Design review of the part shown in the three views and the two pictorial views. Dimensions are in mm from the part's minimum x, y and z. Round coordinates to 2 decimals unless told otherwise and drop trailing zeros. Order: outer loops, then holes, each group sorted by start corner. A loop starts at its lowest first (then second) coordinate and runs counter-clockwise, first axis right, second up. Notation, with made-up numbers: (-23.5, -0.5) - (30.5, -0.5) arc R24 ccw to (30.5, 18.5) - close; hole circle Ø8 at (30, 58). An arc over 180 degrees is marked (long way). Use CSV: the item, a comma, the result in double quotes.
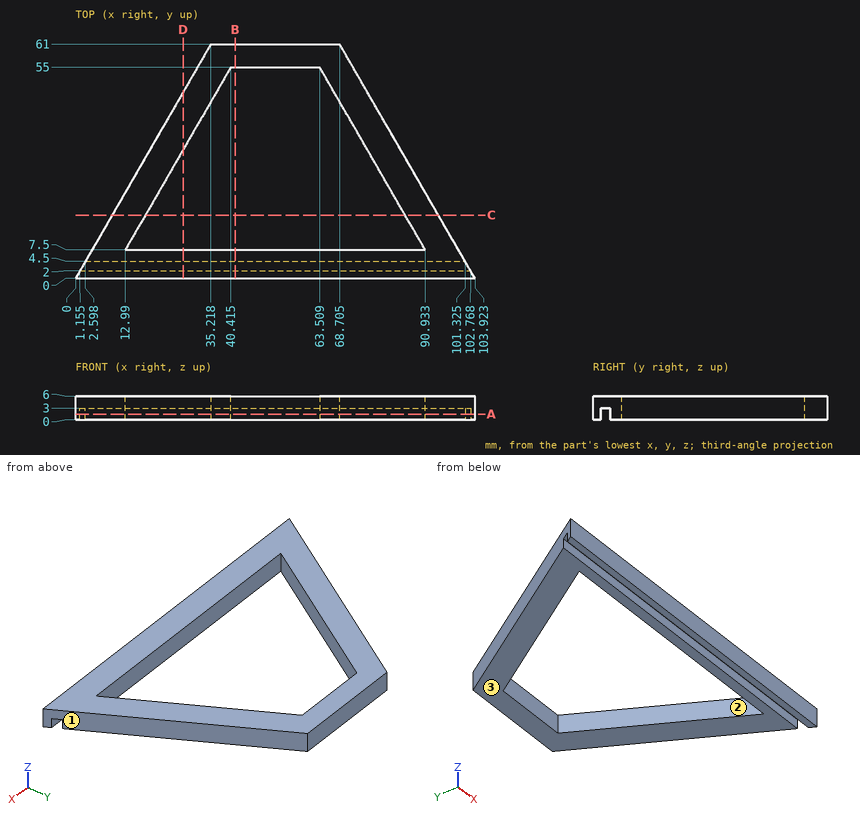
1) We need section B-B (x = 41.5). Give the boundary of the cut face in (y, z).
Data:
outline,"(0, 0) - (2, 0) - (2, 3) - (4.5, 3) - (4.5, 0) - (7.5, 0) - (7.5, 6) - (0, 6) - close; (55, 0) - (61, 0) - (61, 6) - (55, 6) - close"
2) Insertion check: pin 1 Ø2.5 at (x, z) = (27.5, 1.5) entering from +Y (1 decimal); pin 2 Ø8 at (x, y) = (34.5, 29) entering from +Z; pin 3 Ø1.3 at (x, y) = (65.5, 3.5) entering from -Z; pin 4 Ø1 at (y, z) = (54.5, 2.5) entering from -X. Each pin has a flat end and moves straight along its axis. Give the tip position at first contact, or say it passes through.
Data:
pin 1,"stops at y = 49.8"
pin 2,"passes through"
pin 3,"stops at z = 3"
pin 4,"stops at x = 31.18"
3) To check wall thickness, follow L1, parallel to Y at x = 44, z = 2; L2, parallel to Y at x = 63, z = 4.45; L3, parallel to Y at x = 74, z = 0.55 (1 decimal). State the ranges of each line that lie inside material, in increasing order. Write a range as from..to.
Data:
L1,"y = 0..2, 4.5..7.5, 55..61"
L2,"y = 0..7.5, 55..61"
L3,"y = 0..2, 4.5..7.5, 36.8..51.8"
4) We need section C-C (y = 16.5). Give the boundary of the cut face in (x, z), then the cut area to 3 significant figures.
Data:
outline,"(9.53, 0) - (18.19, 0) - (18.19, 6) - (9.53, 6) - close; (85.74, 0) - (94.4, 0) - (94.4, 6) - (85.74, 6) - close"
area,"104 mm2"
5) The part is to be moulded in two halves that separate along Y. For the marked faces 1, 2 and 3, say which applies: +Y half, -Y half, draft (parallel to the pull), parting line (faces both ways), or undercut.
Data:
face 1,"+Y half"
face 2,"undercut"
face 3,"draft"
6) We need section D-D (x = 28). Give the boundary of the cut face in (y, z).
Data:
outline,"(0, 0) - (2, 0) - (2, 3) - (4.5, 3) - (4.5, 0) - (7.5, 0) - (7.5, 6) - (0, 6) - close; (33.5, 0) - (48.5, 0) - (48.5, 6) - (33.5, 6) - close"
7) We need section A-A (z = 1.4). Give the boundary of the cut face in (x, y) (1 decimal), then the cut area to 3 significant figures.
Data:
outline,"(0, 0) - (103.9, 0) - (102.8, 2) - (1.2, 2) - close; (2.6, 4.5) - (101.3, 4.5) - (68.7, 61) - (35.2, 61) - close; hole (13, 7.5) - (90.9, 7.5) - (63.5, 55) - (40.4, 55) - close"
area,"1,540 mm2"
